```python
from build123d import *
from OCP.BRepFilletAPI import BRepFilletAPI_MakeChamfer

# Parameters (mm, degrees)
SALIENTE_EXTRUIR1_DEPTH    = 5
SALIENTE_EXTRUIR2_DEPTH    = 54.34
CORTAR_EXTRUIR1_DEPTH      = 2
CORTAR_EXTRUIR2_DEPTH      = 17
SALIENTE_EXTRUIR3_DEPTH    = 3
SALIENTE_EXTRUIR4_DEPTH    = 15
CROQUIS8_W                 = 19
CROQUIS8_H                 = 5
SALIENTE_EXTRUIR5_DEPTH    = 6
CROQUIS10_R                = 3.375837474
CORTAR_EXTRUIR3_DEPTH      = 10
CROQUIS11_R                = 1.6
CORTAR_EXTRUIR4_DEPTH      = 9
CORTAR_EXTRUIR5_DEPTH      = 138
CORTAR_EXTRUIR5_DEPTH_BACK = 9
CROQUIS12_R                = 3.375837474
CROQUIS13_R                = 4
CORTAR_EXTRUIR6_DEPTH      = 2.2
CROQUIS14_R                = 1.75
CORTAR_EXTRUIR7_DEPTH      = 18.2
CHAFL_N1_SIZE              = 1.75
CHAFL_N1_SIZE2             = 1.631901401
CROQUIS15_W                = 2.505679427
CROQUIS15_H                = 5.945679997
SALIENTE_EXTRUIR6_DEPTH    = 6.2
CROQUIS16_R                = 1.576407793
SALIENTE_EXTRUIR7_DEPTH    = 2.2
REDONDEO1_R                = 10


with BuildPart() as part:
    # Croquis1 → Saliente-Extruir1 (new body)
    with BuildSketch(Plane(origin=(0, 0, 0), x_dir=(1, 0, 0), z_dir=(0, 1, 0))):
        with BuildLine():
            Line((12, 0), (92, 0))
            ThreePointArc((92, 0), (100.485281374, 3.514718626), (104, 12))
            Line((104, 12), (104, 92))
            ThreePointArc((104, 92), (100.485281374, 100.485281374), (92, 104))
            Line((92, 104), (12, 104))
            ThreePointArc((12, 104), (3.514718626, 100.485281374), (0, 92))
            Line((0, 92), (0, 12))
            ThreePointArc((0, 12), (3.514718626, 3.514718626), (12, 0))
        make_face()
    extrude(amount=SALIENTE_EXTRUIR1_DEPTH)

    # Croquis2 → Saliente-Extruir2 (add)
    with BuildSketch(Plane(origin=(0, 5, 0), x_dir=(1, 0, 0), z_dir=(0, 1, 0))):
        with BuildLine():
            Line((12, 0), (92, 0))
            ThreePointArc((92, 0), (100.485281374, 3.514718626), (104, 12))
            Line((104, 12), (104, 92))
            ThreePointArc((104, 92), (100.485281374, 100.485281374), (92, 104))
            Line((92, 104), (12, 104))
            ThreePointArc((12, 104), (3.514718626, 100.485281374), (0, 92))
            Line((0, 92), (0, 12))
            ThreePointArc((0, 12), (3.514718626, 3.514718626), (12, 0))
        make_face()
        with BuildLine():
            Line((12, 3), (92, 3))
            ThreePointArc((92, 3), (98.363961031, 5.636038969), (101, 12))
            Line((101, 12), (101, 92))
            ThreePointArc((101, 92), (98.363961031, 98.363961031), (92, 101))
            Line((92, 101), (12, 101))
            ThreePointArc((12, 101), (5.636038969, 98.363961031), (3, 92))
            Line((3, 92), (3, 12))
            ThreePointArc((3, 12), (5.636038969, 5.636038969), (12, 3))
        make_face(mode=Mode.SUBTRACT)
    extrude(amount=SALIENTE_EXTRUIR2_DEPTH)

    # Croquis3 → Cortar-Extruir1 (cut)
    with BuildSketch(Plane(origin=(0, 59.34, 0), x_dir=(1, 0, 0), z_dir=(0, 1, 0))):
        with BuildLine():
            Line((12, 1.85), (92, 1.85))
            ThreePointArc((92, 1.85), (99.177133829, 4.822866171), (102.15, 12))
            Line((102.15, 12), (102.15, 92))
            ThreePointArc((102.15, 92), (99.177133829, 99.177133829), (92, 102.15))
            Line((92, 102.15), (12, 102.15))
            ThreePointArc((12, 102.15), (4.822866171, 99.177133829), (1.85, 92))
            Line((1.85, 92), (1.85, 12))
            ThreePointArc((1.85, 12), (4.822866171, 4.822866171), (12, 1.85))
        make_face()
    extrude(amount=-CORTAR_EXTRUIR1_DEPTH, mode=Mode.SUBTRACT)

    # Croquis4 → Cortar-Extruir2 (cut)
    with BuildSketch(Plane.XZ):
        with BuildLine():
            Line((23.75, -50.33), (23.75, -58.07))
            ThreePointArc((23.75, -58.07), (26, -64.82), (28.25, -58.07))
            Line((28.25, -58.07), (28.25, -50.33))
            ThreePointArc((28.25, -50.33), (26, -48.08), (23.75, -50.33))
        make_face()
        with BuildLine():
            Line((75.75, -50.33), (75.75, -58.07))
            ThreePointArc((75.75, -58.07), (78, -64.82), (80.25, -58.07))
            Line((80.25, -58.07), (80.25, -50.33))
            ThreePointArc((80.25, -50.33), (78, -48.08), (75.75, -50.33))
        make_face()
    extrude(amount=-CORTAR_EXTRUIR2_DEPTH, mode=Mode.SUBTRACT)

    # Croquis5 → Saliente-Extruir3 (add)
    # profile 1 of 2: a face of its own
    with BuildSketch(Plane(origin=(0, 5, 0), x_dir=(1, 0, 0), z_dir=(0, 1, 0))):
        with BuildLine():
            Line((73.75, 50.33), (73.75, 57.197016654))
            ThreePointArc((73.75, 57.197016654), (78, 66.82), (82.25, 57.197016654))
            Line((82.25, 57.197016654), (82.25, 50.33))
            ThreePointArc((82.25, 50.33), (78, 46.08), (73.75, 50.33))
        make_face()
        with BuildLine():
            Line((80.25, 58.07), (80.25, 50.33))
            ThreePointArc((80.25, 50.33), (78, 48.08), (75.75, 50.33))
            Line((75.75, 50.33), (75.75, 58.07))
            ThreePointArc((75.75, 58.07), (78, 64.82), (80.25, 58.07))
        make_face(mode=Mode.SUBTRACT)
    # profile 2 of 2: a face of its own
    with BuildSketch(Plane(origin=(0, 5, 0), x_dir=(1, 0, 0), z_dir=(0, 1, 0))):
        with BuildLine():
            Line((21.75, 50.33), (21.75, 57.197016654))
            ThreePointArc((21.75, 57.197016654), (26, 66.82), (30.25, 57.197016654))
            Line((30.25, 57.197016654), (30.25, 50.33))
            ThreePointArc((30.25, 50.33), (26, 46.08), (21.75, 50.33))
        make_face()
        with BuildLine():
            Line((23.75, 50.33), (23.75, 58.07))
            ThreePointArc((23.75, 58.07), (26, 64.82), (28.25, 58.07))
            Line((28.25, 58.07), (28.25, 50.33))
            ThreePointArc((28.25, 50.33), (26, 48.08), (23.75, 50.33))
        make_face(mode=Mode.SUBTRACT)
    extrude(amount=SALIENTE_EXTRUIR3_DEPTH)

    # Croquis6 → Saliente-Extruir4 (add)
    with BuildSketch(Plane(origin=(0, 5, 0), x_dir=(1, 0, 0), z_dir=(0, 1, 0))):
        Polygon((14.875650125, 40.19005009), (34.675650125, 40.19005009), (34.675650125, 38.19005009), (32.675650125, 38.19005009), (16.875650125, 38.19005009), (16.875650125, 11.39005009), (32.675650125, 11.39005009), (34.675650125, 11.39005009), (34.675650125, 9.39005009), (14.875650125, 9.39005009), align=None)
    extrude(amount=SALIENTE_EXTRUIR4_DEPTH)

    # Croquis8 → Saliente-Extruir5 (add)
    with BuildSketch(Plane(origin=(0, 5, 0), x_dir=(1, 0, 0), z_dir=(0, 1, 0))):
        with Locations((52, 21.390307978)):
            Rectangle(CROQUIS8_W, CROQUIS8_H)
    saliente_extruir5 = extrude(amount=SALIENTE_EXTRUIR5_DEPTH)

    # Croquis10 → Cortar-Extruir3 (cut)
    with BuildSketch(Plane(origin=(0, 0, -23.890307978), x_dir=(-1, 0, 0), z_dir=(0, 0, -1))):
        with Locations((-52, 11)):
            Circle(CROQUIS10_R)
    cortar_extruir3 = extrude(amount=-CORTAR_EXTRUIR3_DEPTH, mode=Mode.SUBTRACT)

    # Croquis11 → Cortar-Extruir4 (cut)
    with BuildSketch(Plane(origin=(0, 11, 0), x_dir=(1, 0, 0), z_dir=(0, 1, 0))):
        with Locations(Location((58.437918737, 21.390307978, 0), (0, 0, 270))):
            Circle(CROQUIS11_R)
        with Locations(Location((45.562081263, 21.390307978, 0), (0, 0, 90))):
            Circle(CROQUIS11_R)
    cortar_extruir4 = extrude(amount=-CORTAR_EXTRUIR4_DEPTH, mode=Mode.SUBTRACT)

    # Croquis12 → Cortar-Extruir5 (cut, two sides: drawn at the far end of the back side and taken through both)
    with BuildSketch(Plane(origin=(0, 0, -3), x_dir=(-1, 0, 0), z_dir=(0, 0, -1)).offset(-CORTAR_EXTRUIR5_DEPTH_BACK)):
        with Locations((-52, 10)):
            Circle(CROQUIS12_R)
    extrude(amount=CORTAR_EXTRUIR5_DEPTH + CORTAR_EXTRUIR5_DEPTH_BACK, mode=Mode.SUBTRACT)

    # Simetría1: Saliente-Extruir5, Cortar-Extruir3, Cortar-Extruir4 across plane
    add(saliente_extruir5.mirror(Plane(origin=(0, 0, -58.07), x_dir=(1, 0, 0), z_dir=(0, 0, -1))))
    add(cortar_extruir3.mirror(Plane(origin=(0, 0, -58.07), x_dir=(1, 0, 0), z_dir=(0, 0, -1))), mode=Mode.SUBTRACT)
    add(cortar_extruir4.mirror(Plane(origin=(0, 0, -58.07), x_dir=(1, 0, 0), z_dir=(0, 0, -1))), mode=Mode.SUBTRACT)

    # Croquis13 → Cortar-Extruir6 (cut)
    with BuildSketch(Plane.XZ):
        with Locations(Location((72.961798257, -32.537586192, 0), (0, 0, 270))):
            Circle(CROQUIS13_R)
        with Locations(Location((86.181647316, -84.558212342, 0), (0, 0, 270))):
            Circle(CROQUIS13_R)
        with Locations(Location((19.210631353, -84.938725209, 0), (0, 0, 270))):
            Circle(CROQUIS13_R)
    extrude(amount=-CORTAR_EXTRUIR6_DEPTH, mode=Mode.SUBTRACT)

    # Croquis14 → Cortar-Extruir7 (cut)
    with BuildSketch(Plane.XZ.offset(-2.2)):
        with Locations(Location((72.961798257, -32.537586192, 0), (0, 0, 270))):
            Circle(CROQUIS14_R)
        with Locations(Location((86.181647316, -84.558212342, 0), (0, 0, 270))):
            Circle(CROQUIS14_R)
        with Locations(Location((19.210631353, -84.938725209, 0), (0, 0, 270))):
            Circle(CROQUIS14_R)
    extrude(amount=-CORTAR_EXTRUIR7_DEPTH, mode=Mode.SUBTRACT)

    # Chaflán1: one chamfer whose edges measure the first distance from different faces: ONE call of the kernel's chamfer builder (chamfer() names one face for all edges)
    chafl_n1_edges_1 = [part.edges().sort_by_distance(p)[0] for p in [
        (72.961798257, 2.2, -30.787586192),
    ]]
    chafl_n1_side_1 = [part.faces().sort_by_distance(p)[0] for p in [
        (72.961798257, 2.2, -28.650723277),
    ]]
    chafl_n1_edges_2 = [part.edges().sort_by_distance(p)[0] for p in [
        (86.181647316, 2.2, -82.808212342),
    ]]
    chafl_n1_side_2 = [part.faces().sort_by_distance(p)[0] for p in [
        (86.181647316, 2.2, -80.671349427),
    ]]
    chafl_n1_edges_3 = [part.edges().sort_by_distance(p)[0] for p in [
        (19.210631353, 2.2, -83.188725209),
    ]]
    chafl_n1_side_3 = [part.faces().sort_by_distance(p)[0] for p in [
        (19.210631353, 2.2, -81.051862294),
    ]]
    chafl_n1 = BRepFilletAPI_MakeChamfer(part.part.solid().wrapped)
    for e in chafl_n1_edges_1:
        chafl_n1.Add(CHAFL_N1_SIZE, CHAFL_N1_SIZE2, e.wrapped, chafl_n1_side_1[0].wrapped)  # the first distance lies on this face
    for e in chafl_n1_edges_2:
        chafl_n1.Add(CHAFL_N1_SIZE, CHAFL_N1_SIZE2, e.wrapped, chafl_n1_side_2[0].wrapped)  # the first distance lies on this face
    for e in chafl_n1_edges_3:
        chafl_n1.Add(CHAFL_N1_SIZE, CHAFL_N1_SIZE2, e.wrapped, chafl_n1_side_3[0].wrapped)  # the first distance lies on this face
    add(Compound.cast(chafl_n1.Shape()), mode=Mode.REPLACE)

    # Croquis15 → Saliente-Extruir6 (add)
    with BuildSketch(Plane(origin=(0, 5, 0), x_dir=(1, 0, 0), z_dir=(0, 1, 0))):
        with Locations((31.675296524, 28.865498451)):
            Rectangle(CROQUIS15_W, CROQUIS15_H)
    extrude(amount=SALIENTE_EXTRUIR6_DEPTH)

    # Croquis16 → Saliente-Extruir7 (add)
    with BuildSketch(Plane(origin=(0, 5, 0), x_dir=(1, 0, 0), z_dir=(0, 1, 0))):
        with BuildLine():
            ThreePointArc((20.979111053, 13.100030069), (19.317879756, 14.761261366), (17.656648458, 13.100030069))
            Line((17.656648458, 13.100030069), (17.656648458, 11.39005009))
            Line((17.656648458, 11.39005009), (20.979111053, 11.39005009))
            Line((20.979111053, 11.39005009), (20.979111053, 13.100030069))
        make_face()
        with Locations(Location((28.220818392, 23.4710535, 0), (0, 0, 90))):
            Circle(CROQUIS16_R)
        with BuildLine():
            Line((24.185453679, 38.19005009), (24.185453679, 36.107269041))
            ThreePointArc((24.185453679, 36.107269041), (25.888394883, 34.404327838), (27.591336086, 36.107269041))
            Line((27.591336086, 36.107269041), (27.591336086, 38.19005009))
            Line((27.591336086, 38.19005009), (24.185453679, 38.19005009))
        make_face()
    extrude(amount=SALIENTE_EXTRUIR7_DEPTH)

    # Redondeo1
    redondeo1_edges = [part.edges().sort_by_distance(p)[0] for p in [
        (34.675650125, 20, -39.19005009),
        (34.675650125, 20, -10.39005009),
    ]]
    fillet(redondeo1_edges, radius=REDONDEO1_R)


solid = part.part
```
CAD build for the part. Positions are in the model's coordinates, mm. A direction names the side the tool comes from. Round coordinates to 2 decimals unless told otherwise and drop trailing zeros. Order: outer loops, then holes, each group sorted by start corner. A loop starts at its lowest first (then second) coordinate and runs counter-clockwise, first axis right, second up. Notation, with made-up numbers: (38.25, -14.75) - (92.25, -14.75) arc R24 cw to (92.25, -1.75) - close; hole circle Ø9 at (-17, 74.5). An arc over 180 degrees is marked (long way). Answer in a Markdown table with one row per item. Add a question column.
(1) Band-saw the part on C-C on x = 95.5. List the corners of the cut face in (y, z), and give its area (3 significant figures).
(2) Band-saw the part on B-B on y = 34. List the corners of the cut face in (x, z).
(3) Band-saw the part on A-A on z = -61.07. List the corners of the cut face in (x, y), and give its area (3 significant figures).
(4) 3-axis set-ups, long thin cutter, end or side, ignore diameter. For faces 1 (the face through (17, 2.2, -88)), 2 (the face through (25, 12, -40.19)), 3 (the face through (52.081, 6.625, -21.355)): which of +Z, -Z, +X, -X, +Y, -Y reach the whole face in a straight line?
(5) Probe L1, parallel to X at y = 49.5, z = -26; L2, parallel to Z at x = 50.5, y = 21.5; L3, parallel to Y at x = 68.5, z = -16. List the from-to ranges inside material, lowest first. Write a range as [from, to].
(6) Drop flat-ended pins along their axis: pin 1 Ø5 at (x, z) = (19.5, -26.5) entering from +Y; pin 2 Ø10 at (x, z) = (82, -68.5) entering from +Y; pin 3 Ø2 at (x, z) = (44, -23.5) entering from +Y. Give the stop position or say it passes through.
(7) Mould opens along X. For faces 4 (the face through (32.5, 59.34, -102.32)), 5 (the face through (104, 29, -51)), 6 (the face through (30.25, 6, -54)) say: +X half, -X half, draft (parallel to the pull), parting line (faces both ways), or undercut.
(8) Band-saw the part on D-D on z = -42. List the corners of the cut face in (x, y), and give its area (3 significant figures).
Data:
| question | item | result |
|---|---|---|
| 1 | outline | (0, -103.48) - (59.34, -103.48) - (59.34, -101.53) - (57.34, -101.53) - (57.34, -100.29) - (5, -100.29) - (5, -3.71) - (57.34, -3.71) - (57.34, -2.47) - (59.34, -2.47) - (59.34, -0.52) - (0, -0.52) - close |
| 1 | area | 856 mm^2 |
| 2 | outline | (0, -92) arc R12 ccw to (12, -104) - (92, -104) arc R12 ccw to (104, -92) - (104, -12) arc R12 ccw to (92, 0) - (12, 0) arc R12 ccw to (0, -12) - close; hole (3, -92) arc R9 ccw to (12, -101) - (92, -101) arc R9 ccw to (101, -92) - (101, -12) arc R9 ccw to (92, -3) - (12, -3) arc R9 ccw to (3, -12) - close |
| 3 | outline | (0, 0) - (22.25, 0) - (22.25, 8) - (20.25, 8) - (20.25, 5) - (3, 5) - (3, 57.34) - (1.85, 57.34) - (1.85, 59.34) - (0, 59.34) - close; (29.75, 0) - (74.25, 0) - (74.25, 8) - (72.25, 8) - (72.25, 5) - (31.75, 5) - (31.75, 8) - (29.75, 8) - close; (81.75, 0) - (104, 0) - (104, 59.34) - (102.15, 59.34) - (102.15, 57.34) - (101, 57.34) - (101, 5) - (83.75, 5) - (83.75, 8) - (81.75, 8) - close |
| 3 | area | 790 mm^2 |
| 4 | face 1 | -Y |
| 4 | face 2 | +Y |
| 4 | face 3 | +Z |
| 5 | L1 | x = [0, 3], [101, 104] |
| 5 | L2 | z = [-104, -101], [-3, 0] |
| 5 | L3 | y = [0, 5] |
| 6 | pin 1 | stops at y = 5 |
| 6 | pin 2 | stops at y = 8 |
| 6 | pin 3 | stops at y = 11 |
| 7 | face 4 | draft |
| 7 | face 5 | +X half |
| 7 | face 6 | undercut |
| 8 | outline | (0, 0) - (104, 0) - (104, 59.34) - (102.15, 59.34) - (102.15, 57.34) - (101, 57.34) - (101, 5) - (3, 5) - (3, 57.34) - (1.85, 57.34) - (1.85, 59.34) - (0, 59.34) - close |
| 8 | area | 841 mm^2 |
